```python
from build123d import *


with BuildPart() as f1:
    # F0 (on Right) → F1 (revolve)
    with BuildSketch(Plane.YZ):
        Polygon((-25, 11.278154), (-25, 12.082125), (-28, 11.278154), align=None)
        with BuildLine():
            Line((0, 0), (0, 20.5))
            Line((0, 20.5), (-28.65, 20.5))
            ThreePointArc((-28.65, 20.5), (-29.71066, 20.06066), (-30.15, 19))
            Line((-30.15, 19), (-30.15, 17))
            Line((-30.15, 17), (-25, 17))
            Line((-25, 17), (-25, 12.082125))
            Line((-25, 12.082125), (-25, 11.278154))
            Line((-25, 11.278154), (-25, 9.414572))
            Line((-25, 9.414572), (-25, 8.610601))
            Line((-25, 8.610601), (-25, 7.80663))
            Line((-25, 7.80663), (-25, 5.943048))
            Line((-25, 5.943048), (-25, 5.139077))
            Line((-25, 5.139077), (-25, 4.335106))
            Line((-25, 4.335106), (-25, 2.471524))
            Line((-25, 2.471524), (-25, 0))
            Line((-25, 0), (0, 0))
        make_face()
        Polygon((-28, 4.335106), (-25, 2.471524), (-25, 4.335106), align=None)
        Polygon((-28, 7.80663), (-25, 7.80663), (-25, 8.610601), align=None)
        Polygon((-25, 9.414572), (-25, 11.278154), (-28, 11.278154), align=None)
        Polygon((-28, 4.335106), (-25, 4.335106), (-25, 5.139077), align=None)
        Polygon((-28, 7.80663), (-25, 5.943048), (-25, 7.80663), align=None)
    revolve(axis=Axis((0, 0, 10.25), (0, 0, 1)))


solid = f1.part
```
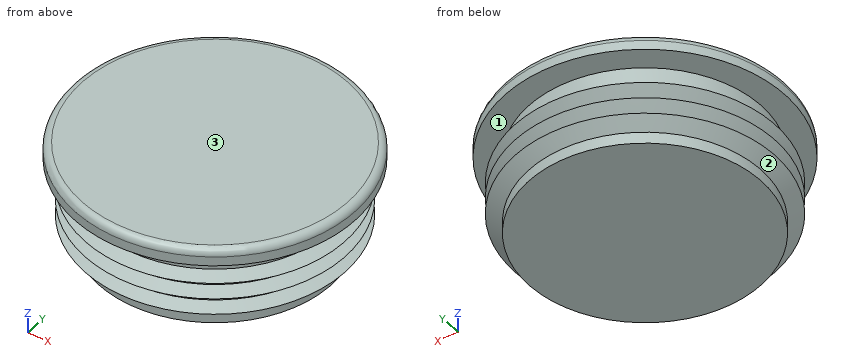
Here's how the part is built. I have some questions about the finished solid (model axes, mm). Face numbers are marked on the shaded views. Coordinates: 2 decimals unless noted, no trailing zeros. Loops run counter-clockwise (first coordinate to the right, second up) from the corner with the lowest first, then second, coordinate; pieces in that order, holes last. Notation, with made-up numbers: (51, -11.5) - (77, -11.5) arc R24 ccw to (77, 0.5) - close; hole circle Ø8 at (82, -15.5). An arc over 180 degrees is marked (long way). Return JSON: item names as keys, results as strings. Group by question number.
Item 1: If we section it at D-D on z = 1.75: Write out the boundary of the cut face in (x, y).
Item 2: If we section it at A-A on x = 0: Write out the boundary of the cut face in (y, z), and give its area (3 significant figures).
Item 3: Will these pins go through, and if not, where does the flat tip stop? P1, Ø12, axis at x = -13, z = 12, coming from the +Y side; P2, Ø6, axis at x = 21.5, y = 19.5, coming from the -Z side; P3, Ø3, axis at y = 11, z = 16.5, coming from the -X side; P4, Ø12, axis at x = 20, y = -5.5, coming from the -Z side.
Item 4: We'd pull the mould along Z, two halves only. Please class the marked faces 1, 2 and 3: +Z half, -Z half, draft (parallel to the pull), parting line (faces both ways), or undercut.
Item 5: I need wall thicknesses on line 1 (Z direction, x = -24.5, y = 13); line 2 (Z direction, x = 17.5, y = 20.5); line 3 (Z direction, x = 14, y = -25). Which ranges of each line are inside material? Lowest first, please. Write a range as from..to.
Item 6: If we section it at C-C on y = -26: State how many separate pieces and enclosed holes the cut face has, and give its area (3 significant figures).
Calculated:
{
 "1": {"outline": "circle Ø50 at (0, 0)"},
 "2": {"outline": "(-30.15, 17) - (-25, 17) - (-25, 12.08) - (-28, 11.28) - (-25, 9.41) - (-25, 8.61) - (-28, 7.81) - (-25, 5.94) - (-25, 5.14) - (-28, 4.34) - (-25, 2.47) - (-25, 0) - (25, 0) - (25, 2.47) - (28, 4.34) - (25, 5.14) - (25, 5.94) - (28, 7.81) - (25, 8.61) - (25, 9.41) - (28, 11.28) - (25, 12.08) - (25, 17) - (30.15, 17) - (30.15, 19) arc R1.5 ccw to (28.65, 20.5) - (-28.65, 20.5) arc R1.5 ccw to (-30.15, 19) - close", "area": "1,080 mm^2"},
 "3": {"P1": "stops at y = 28.55", "P2": "stops at z = 3.11", "P3": "stops at x = -28.59", "P4": "stops at z = 0"},
 "4": {"face 1": "undercut", "face 2": "-Z half", "face 3": "+Z half"},
 "5": {"line 1": "z = 4.17..4.41, 7.64..7.88, 11.11..11.35, 17..20.5", "line 2": "z = 3.69..4.62, 7.16..8.09, 10.63..11.56, 17..20.5", "line 3": "z = 17..20.5"},
 "6": {"separate pieces": "4", "enclosed holes": "0", "area": "178 mm^2"}
}
